Here's how the part is built. I have some questions about the finished solid (model axes, mm). A direction names the side the tool comes from. Give positions to 0.01 mm unless a question says otherwise; leave off trailing zeros. Write each loop counter-clockwise with the first axis right and the second up, starting at its lowest first coordinate (ties: lowest second). Pieces come first, ordered by that corner, then holes. Notation, with made-up numbers: (87.25, -23.75) - (126.25, -23.75) arc R7 ccw to (126.25, -14.75) - close; hole circle Ø2 at (-29.75, 12). An arc over 180 degrees is marked (long way). One line per item, written item: value. Start each with the question number.
1) Imagine slicing it at B-B on y = -6. Write out the boundary of the cut face in (x, z).
2) Please list where these lines run through material, in increasing order: L1, parallel to Y at x = 25.75, z = 17.55; L2, parallel to X at y = -3.25, z = 29; L3, parallel to Z at x = 18, y = -6.25. Write a range as [from, to].
3) Imagine slicing it at A-A on x = 25.75. Write out the boundary of the cut face in (y, z), plus the area to 3 significant figures.
4) Imagine slicing it at C-C on z = 24. Write out the boundary of the cut face in (x, y), plus the area to 3 significant figures.
5) We'd pull the mould along Y, two halves only. Please class faces 4 (the cylindrical face through (3.252, -5.912, 31.972)), 5 (the flat face through (23.7, -5.9, 16)), 6 (the cylindrical face through (6.54, -6.54, 16.76)): +Y half, -Y half, draft (parallel to the pull), parting line (faces both ways), or undercut.
6) Imagine slicing it at D-D on x = 5.25. Write out the boundary of the cut face in (y, z), plus the area to 3 significant figures.
7) I'm going to push flat-ended pins straight in: P1, Ø3.5, axis at x = 26, y = -4, coming from the -Z side; P2, Ø4.5, axis at x = 26, y = -5, coming from the +Z side; P3, Ø3, axis at x = 20.5, y = -3.5, coming from the +Z side; P4, Ø2, axis at x = -2.25, y = -6, coming from the +Z side (3 decimals). Where does each tip first touch, or does it pass through?
8) On a 3-axis mill with a long thin cutter (end or side, diameter ignored), from which of +Z, -Z, +X, -X, +Y, -Y can I reach the whole of each face in a straight line? I mean faces 1 (the flat face through (23.5, -6, 8)), 2 (the flat face through (-0.3, -5.9, 16)), 3 (the flat face through (23.8, -5.9, 18)). Say none if no direction works.
from build123d import *

# Parameters (mm, degrees)
PAD019_DEPTH      = 12
SKETCH028_R       = 1.65
POCKET008_DEPTH   = 50
CYLINDER_R        = 2
CYLINDER_DEPTH    = 34
CYLINDER001_R     = 1.4
CYLINDER001_DEPTH = 34


with BuildPart() as part:
    # Sketch027 → Pad019 (new body)
    with BuildSketch(Plane.XZ):
        Polygon((0, 0), (23.5, 0), (23.5, 16), (27.75, 16), (27.75, 18), (23.5, 18), (23.5, 30), (0, 30), (0, 18), (-4.25, 18), (-4.25, 16), (0, 16), align=None)
    extrude(amount=PAD019_DEPTH)

    # Sketch028 → Pocket008 (cut)
    with BuildSketch(Plane.XY):
        with Locations((-2.25, -6)):
            Circle(SKETCH028_R)
        with Locations((25.75, -6)):
            Circle(SKETCH028_R)
    extrude(amount=POCKET008_DEPTH, mode=Mode.SUBTRACT)

    # Cylinder → Cylinder (join)
    with BuildSketch(Plane(origin=(5.25, -6, 0), x_dir=(1, 0, 0), z_dir=(0, 0, 1))):
        Circle(CYLINDER_R)
    extrude(amount=CYLINDER_DEPTH)

    # Cylinder001 → Cylinder001 (cut)
    with BuildSketch(Plane(origin=(5.25, -6, 0), x_dir=(1, 0, 0), z_dir=(0, 0, 1))):
        Circle(CYLINDER001_R)
    extrude(amount=CYLINDER001_DEPTH, mode=Mode.SUBTRACT)


solid = part.part
Numbers:
1. outline: (-4.25, 16) - (-3.9, 16) - (-3.9, 18) - (-4.25, 18) - close; (-0.6, 16) - (0, 16) - (0, 0) - (3.85, 0) - (3.85, 34) - (3.25, 34) - (3.25, 30) - (0, 30) - (0, 18) - (-0.6, 18) - close; (6.65, 0) - (23.5, 0) - (23.5, 16) - (24.1, 16) - (24.1, 18) - (23.5, 18) - (23.5, 30) - (7.25, 30) - (7.25, 34) - (6.65, 34) - close; (27.4, 16) - (27.75, 16) - (27.75, 18) - (27.4, 18) - close
2. L1: [-12, -7.65], [-4.35, 0]
2. L2: [0, 23.5]
2. L3: [0, 30]
3. outline: (-12, 16) - (-7.65, 16) - (-7.65, 18) - (-12, 18) - close; (-4.35, 16) - (0, 16) - (0, 18) - (-4.35, 18) - close
3. area: 17.4 mm^2
4. outline: (0, -12) - (23.5, -12) - (23.5, 0) - (0, 0) - close; hole circle Ø2.8 at (5.25, -6)
4. area: 276 mm^2
5. face 4: parting line
5. face 5: draft
5. face 6: undercut
6. outline: (-12, 0) - (-7.4, 0) - (-7.4, 34) - (-8, 34) - (-8, 30) - (-12, 30) - close; (-4.6, 0) - (0, 0) - (0, 30) - (-4, 30) - (-4, 34) - (-4.6, 34) - close
6. area: 281 mm^2
7. P1: z = 16
7. P2: z = 18
7. P3: z = 30
7. P4: through
8. face 1: -Z, +X, +Y, -Y
8. face 2: -Z, -X, +Y, -Y
8. face 3: +Z, +X, +Y, -Y
